from build123d import *

# Parameters (mm, degrees)
SKETCH1_W           = 430
SKETCH1_H           = 110
SKETCH1_W_2         = 400
SKETCH1_H_2         = 80
BOSS_EXTRUDE1_DEPTH = 80
SKETCH2_W           = 430
SKETCH2_H           = 110
BOSS_EXTRUDE2_DEPTH = 10
SKETCH3_R           = 21
CUT_EXTRUDE1_DEPTH  = 196
FILLET1_R           = 5
CIRPATTERN1_COUNT   = 6
CIRPATTERN2_COUNT   = 6
CIRPATTERN3_COUNT   = 6


with BuildPart() as part:
    # Sketch1 → Boss-Extrude1 (new body)
    with BuildSketch(Plane(origin=(0, 0, 0), x_dir=(1, 0, 0), z_dir=(0, 1, 0))):
        Rectangle(SKETCH1_W, SKETCH1_H)
        Rectangle(SKETCH1_W_2, SKETCH1_H_2, mode=Mode.SUBTRACT)
    extrude(amount=BOSS_EXTRUDE1_DEPTH)

    # Sketch2 → Boss-Extrude2 (add)
    with BuildSketch(Plane(origin=(0, 80, 0), x_dir=(1, 0, 0), z_dir=(0, 1, 0))):
        Rectangle(SKETCH2_W, SKETCH2_H)
    extrude(amount=BOSS_EXTRUDE2_DEPTH)

    # Sketch3 → Cut-Extrude1 (cut)
    with BuildSketch(Plane.XY.offset(55)):
        with Locations((135, 0)):
            Circle(SKETCH3_R)
        with Locations((43, 0)):
            Circle(SKETCH3_R)
        with Locations((-85, 0)):
            Circle(SKETCH3_R)
    extrude(amount=-CUT_EXTRUDE1_DEPTH, mode=Mode.SUBTRACT)

    # Fillet1
    fillet1_edges = [part.edges().sort_by_distance(p)[0] for p in [
        (200, 40, 40),
        (200, 40, -40),
        (-200, 40, -40),
        (-200, 40, 40),
        (200, 80, 0),
        (0, 80, -40),
        (-200, 80, 0),
        (0, 80, 40),
        (215, 90, 0),
        (0, 90, -55),
        (-215, 90, 0),
        (0, 90, 55),
        (215, 45, 55),
        (-215, 45, 55),
        (-215, 45, -55),
        (215, 45, -55),
    ]]
    fillet(fillet1_edges, radius=FILLET1_R)

    # Sketch6 → M5 Tapped Hole1 (revolve, cut)
    with BuildSketch(Plane(origin=(158.815698604, 13.75, -55), x_dir=(0, 1, 0), z_dir=(1, 0, 0))):
        Polygon((0, 0), (0, 13.6618073), (2.1, 12.4), (2.1, 0.425), (2.525, 0), align=None)
    m5_tapped_hole1 = revolve(axis=Axis((158.815698604, 13.75, -61.35), (0, 0, 1)), mode=Mode.SUBTRACT)

    # Sketch7 → M5 Tapped Hole2 (revolve, cut)
    with BuildSketch(Plane(origin=(66.815698604, 13.75, -55), x_dir=(0, 1, 0), z_dir=(1, 0, 0))):
        Polygon((0, 0), (0, 13.6618073), (2.1, 12.4), (2.1, 0.425), (2.525, 0), align=None)
    m5_tapped_hole2 = revolve(axis=Axis((66.815698604, 13.75, -61.35), (0, 0, 1)), mode=Mode.SUBTRACT)

    # Sketch10 → M5 Tapped Hole3 (revolve, cut)
    with BuildSketch(Plane(origin=(-61.184301396, 13.75, -55), x_dir=(0, 1, 0), z_dir=(1, 0, 0))):
        Polygon((0, 0), (0, 13.6618073), (2.1, 12.4), (2.1, 0.425), (2.525, 0), align=None)
    m5_tapped_hole3 = revolve(axis=Axis((-61.184301396, 13.75, -61.35), (0, 0, 1)), mode=Mode.SUBTRACT)

    # CirPattern1: M5 Tapped Hole1 ×6 about axis, 3 skipped
    cirpattern1_axis = Axis((135, 0, 0), (0, 0, 1))
    add([m5_tapped_hole1.rotate(cirpattern1_axis, i * 360 / CIRPATTERN1_COUNT) for i in range(1, CIRPATTERN1_COUNT) if i not in (3, 4, 5)], mode=Mode.SUBTRACT)

    # CirPattern2: M5 Tapped Hole2 ×6 about axis, 3 skipped
    cirpattern2_axis = Axis((43, 0, -141), (0, 0, -1))
    add([m5_tapped_hole2.rotate(cirpattern2_axis, i * 360 / CIRPATTERN2_COUNT) for i in range(1, CIRPATTERN2_COUNT) if i not in (1, 2, 3)], mode=Mode.SUBTRACT)

    # CirPattern3: M5 Tapped Hole3 ×6 about axis, 3 skipped
    cirpattern3_axis = Axis((-85, 0, 0), (0, 0, 1))
    add([m5_tapped_hole3.rotate(cirpattern3_axis, i * 360 / CIRPATTERN3_COUNT) for i in range(1, CIRPATTERN3_COUNT) if i not in (3, 4, 5)], mode=Mode.SUBTRACT)

    # Mirror1: M5 Tapped Hole1, M5 Tapped Hole2, M5 Tapped Hole3 across plane
    add(m5_tapped_hole1.mirror(Plane.XY), mode=Mode.SUBTRACT)
    add(m5_tapped_hole2.mirror(Plane.XY), mode=Mode.SUBTRACT)
    add(m5_tapped_hole3.mirror(Plane.XY), mode=Mode.SUBTRACT)

    # Mirror1 copy 1 sketch → Mirror1 copy 1 (revolve, cut)
    with BuildSketch(Plane(origin=(135, 27.5, 55), x_dir=(-0.866025404, 0.5, 0), z_dir=(0.5, 0.866025404, 0))):
        Polygon((0, 0), (0, -13.6618073), (2.1, -12.4), (2.1, -0.425), (2.525, 0), align=None)
    revolve(axis=Axis((135, 27.5, 61.35), (0, 0, 1)), mode=Mode.SUBTRACT)

    # Mirror1 copy 2 sketch → Mirror1 copy 2 (revolve, cut)
    with BuildSketch(Plane(origin=(111.184301396, 13.75, 55), x_dir=(-0.866025404, -0.5, 0), z_dir=(-0.5, 0.866025404, 0))):
        Polygon((0, 0), (0, -13.6618073), (2.1, -12.4), (2.1, -0.425), (2.525, 0), align=None)
    revolve(axis=Axis((111.184301396, 13.75, 61.35), (0, 0, 1)), mode=Mode.SUBTRACT)

    # Mirror1 copy 3 sketch → Mirror1 copy 3 (revolve, cut)
    with BuildSketch(Plane(origin=(19.184301396, 13.75, 55), x_dir=(-0.866025404, -0.5, 0), z_dir=(-0.5, 0.866025404, 0))):
        Polygon((0, 0), (0, -13.6618073), (2.1, -12.4), (2.1, -0.425), (2.525, 0), align=None)
    revolve(axis=Axis((19.184301396, 13.75, 61.35), (0, 0, 1)), mode=Mode.SUBTRACT)

    # Mirror1 copy 4 sketch → Mirror1 copy 4 (revolve, cut)
    with BuildSketch(Plane(origin=(43, 27.5, 55), x_dir=(-0.866025404, 0.5, 0), z_dir=(0.5, 0.866025404, 0))):
        Polygon((0, 0), (0, -13.6618073), (2.1, -12.4), (2.1, -0.425), (2.525, 0), align=None)
    revolve(axis=Axis((43, 27.5, 61.35), (0, 0, 1)), mode=Mode.SUBTRACT)

    # Mirror1 copy 5 sketch → Mirror1 copy 5 (revolve, cut)
    with BuildSketch(Plane(origin=(-85, 27.5, 55), x_dir=(-0.866025404, 0.5, 0), z_dir=(0.5, 0.866025404, 0))):
        Polygon((0, 0), (0, -13.6618073), (2.1, -12.4), (2.1, -0.425), (2.525, 0), align=None)
    revolve(axis=Axis((-85, 27.5, 61.35), (0, 0, 1)), mode=Mode.SUBTRACT)

    # Mirror1 copy 6 sketch → Mirror1 copy 6 (revolve, cut)
    with BuildSketch(Plane(origin=(-108.815698604, 13.75, 55), x_dir=(-0.866025404, -0.5, 0), z_dir=(-0.5, 0.866025404, 0))):
        Polygon((0, 0), (0, -13.6618073), (2.1, -12.4), (2.1, -0.425), (2.525, 0), align=None)
    revolve(axis=Axis((-108.815698604, 13.75, 61.35), (0, 0, 1)), mode=Mode.SUBTRACT)


solid = part.part
For this review, take the finished solid that the model builds, in its own axes (mm). A direction names the side the tool comes from. Coordinates: 2 decimals unless noted, no trailing zeros. Write each loop counter-clockwise with the first axis right and the second up, starting at its lowest first coordinate (ties: lowest second). Pieces come first, ordered by that corner, then holes. Notation, with made-up numbers: (34.25, 50.25) -> (40.25, 50.25) arc R22 ccw to (40.25, 83.25) -> close; hole circle Ø9 at (-13, 47). An arc over 180 degrees is marked (long way). Write each question's results on one line, items separated by ' | '. Start each with the question number.
1) Consider section B-B (y = 38). Write out the cut boundary in (x, z).
2) The part is to be moulded in two halves that separate along Z. For faces 3 (the face through (-215, 42, 1)), 4 (the face through (200, 37, 0)), 5 (the face through (-3, 42, 55)), 6 (the face through (-3, 37, -40)), say which applies: +Z half, -Z half, draft (parallel to the pull), parting line (faces both ways), or undercut.
3) Consider section C-C (z = 16). Write out the cut boundary in (x, y).
4) Wall thickness on L1, parallel to Z at x = 41, y = 41.5; L2, parallel to X at y = 22.5, z = 18; L3, parallel to Y at x = 43, z = -47: over which ranges is each line inside the solid? List them lowest first. Write a range as [from, to].
5) For faces 1 (the face through (-3, 80, 0)), 2 (the face through (-22, 0, -48)), list the 3-axis set-ups (+Z, -Z, +X, -X, +Y, -Y) from which the entire face can be reached by the end or side of a thin tool; tool diameter is ignored.
6) Insertion check: pin 1 (5.5 mm diameter, centred on x = 135, y = 27.5, fed in from -Z); pin 2 (3.5 mm diameter, centred on x = 66.82, y = 13.75, fed in from +Z); pin 3 (4 mm diameter, centred on x = 43, y = 27.5, fed in from +Z); pin 4 (2.5 mm diameter, centred on x = -85, y = 27.5, fed in from +Z). Each pin has a flat end and moves straight along its axis. Give the tip position at first contact, or say it passes through.
7) Consider section A-A (x = -38.5). Write out the cut boundary in (y, z).
Geometry says:
1) outline: (-215, -50) arc R5 ccw to (-210, -55) -> (210, -55) arc R5 ccw to (215, -50) -> (215, 50) arc R5 ccw to (210, 55) -> (-210, 55) arc R5 ccw to (-215, 50) -> close; hole (-200, -35) arc R5 ccw to (-195, -40) -> (195, -40) arc R5 ccw to (200, -35) -> (200, 35) arc R5 ccw to (195, 40) -> (-195, 40) arc R5 ccw to (-200, 35) -> close
2) face 3: draft | face 4: undercut | face 5: +Z half | face 6: undercut
3) outline: (-215, 0) -> (-200, 0) -> (-200, 75) arc R5 cw to (-195, 80) -> (195, 80) arc R5 cw to (200, 75) -> (200, 0) -> (215, 0) -> (215, 85) arc R5 ccw to (210, 90) -> (-210, 90) arc R5 ccw to (-215, 85) -> close
4) L1: [-55, -40], [40, 55] | L2: [-215, -200], [200, 215] | L3: [21, 25.4], [29.6, 90]
5) face 1: -Y | face 2: +Z, -Z, +X, -X, -Y
6) pin 1: z = -55 | pin 2: z = 42.39 | pin 3: z = 42.54 | pin 4: z = 42.09
7) outline: (0, -55) -> (85, -55) arc R5 ccw to (90, -50) -> (90, 50) arc R5 ccw to (85, 55) -> (0, 55) -> (0, 40) -> (75, 40) arc R5 cw to (80, 35) -> (80, -35) arc R5 cw to (75, -40) -> (0, -40) -> close
